from build123d import *

# Parameters (mm, degrees)
SKETCH1_R                  = 6.4
BOSS_EXTRUDE1_DEPTH        = 66.73
F_10_24_TAPPED_HOLE1_D     = 3.7973
F_10_24_TAPPED_HOLE1_DEPTH = 12.83
F_10_24_TAPPED_HOLE1_TIP   = 1.140824014
F_10_24_TAPPED_HOLE2_D     = 3.7973
F_10_24_TAPPED_HOLE2_DEPTH = 12.83
F_10_24_TAPPED_HOLE2_TIP   = 1.140824014


with BuildPart() as part:
    # Sketch1 → Boss-Extrude1 (new body)
    with BuildSketch(Plane.XY):
        Circle(SKETCH1_R)
    extrude(amount=BOSS_EXTRUDE1_DEPTH)

    # #10-24 Tapped Hole1
    with Locations(Plane(origin=(0, 0, 0), x_dir=(-1, 0, 0), z_dir=(0, 0, -1))):
        with Locations((0, 0)):
            Hole(F_10_24_TAPPED_HOLE1_D / 2, depth=F_10_24_TAPPED_HOLE1_DEPTH)
            with Locations((0, 0, -(F_10_24_TAPPED_HOLE1_DEPTH + F_10_24_TAPPED_HOLE1_TIP / 2))):  # 118° drill point
                Cone(0, F_10_24_TAPPED_HOLE1_D / 2, F_10_24_TAPPED_HOLE1_TIP, mode=Mode.SUBTRACT)

    # #10-24 Tapped Hole2
    with Locations(Plane.XY.offset(66.73)):
        with Locations((0, 0)):
            Hole(F_10_24_TAPPED_HOLE2_D / 2, depth=F_10_24_TAPPED_HOLE2_DEPTH)
            with Locations((0, 0, -(F_10_24_TAPPED_HOLE2_DEPTH + F_10_24_TAPPED_HOLE2_TIP / 2))):  # 118° drill point
                Cone(0, F_10_24_TAPPED_HOLE2_D / 2, F_10_24_TAPPED_HOLE2_TIP, mode=Mode.SUBTRACT)


solid = part.part
CAD build for the part. Positions are in the model's coordinates, mm. A direction names the side the tool comes from. Give positions to 0.01 mm unless a question says otherwise; leave off trailing zeros. Order: outer loops, then holes, each group sorted by start corner. A loop starts at its lowest first (then second) coordinate and runs counter-clockwise, first axis right, second up. Notation, with made-up numbers: (46, -33.5) -> (76, -33.5) arc R12 ccw to (76, -25.5) -> close; hole circle Ø9 at (-35, -5). An arc over 180 degrees is marked (long way). Return JSON: item names as keys, results as strings.
Q1. Drill centre lines: line 1 (Y direction, x = 0, z = 8.75); line 2 (X direction, y = -0.5, z = 56.5); line 3 (X direction, y = 5.5, z = 24). Where is each one in solid material? Low to high.
Working result:
{"line 1": "-6.4 to -1.9, 1.9 to 6.4", "line 2": "-6.38 to -1.83, 1.83 to 6.38", "line 3": "-3.27 to 3.27"}
Q2. Which spindle directions (+Z, -Z, +X, -X, +Y, -Y) get a long thin tool onto all of the face, cutting with end or side? Do faces 5 (the face through (1, 2, 66.73)), 6 (the face through (-1.8, 0.6, 60.2)), 7 (the face through (1.8, 0.6, 6.5)). Say none if no direction does.
Working result:
{"face 5": "+Z, +X, -X, +Y, -Y", "face 6": "+Z", "face 7": "-Z"}
Q3. Saw through at B-B (z = 39). Write the cut outline in (x, y).
Working result:
{"outline": "circle Ø12.8 at (0, 0)"}
Q4. Mould opens along X. For faces 1 (the face through (1, 2, 0)), 2 (the face through (-5.08, -3.89, 32.9)), 3 (the face through (0.315, 0.099, 52.957)), 4 (the face through (-0.18, 0.28, 13.77)) say: pulls with the +X half, pulls with the -X half, needs draft (parallel to the pull), parting line crosses it, or undercut.
Working result:
{"face 1": "needs draft", "face 2": "parting line crosses it", "face 3": "undercut", "face 4": "undercut"}
Q5. Flat gauge pins, fed straight in: pin 1 (5 mm diameter, centred on x = 4, z = 55, fed in from -Y); pin 2 (1 mm diameter, centred on y = -4.5, z = 53, fed in from -X); pin 3 (2.5 mm diameter, centred on x = 0, y = 0, fed in from +Z). Where does each tip first touch, or does it go through?
Working result:
{"pin 1": "y = -6.22", "pin 2": "x = -5", "pin 3": "z = 53.51"}
Q6. Saw through at C-C (x = 4). Write the cut outline in (y, z), then the cut area to 3 significant figures.
Working result:
{"outline": "(-5, 0) -> (5, 0) -> (5, 66.73) -> (-5, 66.73) -> close", "area": "667 mm²"}
Q7. Saw through at A-A (z = 58). Write the cut outline in (x, y).
Working result:
{"outline": "circle Ø12.8 at (0, 0); hole circle Ø3.8 at (0, 0)"}
